Autodesk Inventor part; units mm, degrees
ref_plane "YZ Plane" through (0, 0, 0) normal (1, 0, 0) x (0, 1, 0)
ref_plane "XZ Plane" through (0, 0, 0) normal (0, 1, 0) x (-1, 0, 0)
ref_plane "XY Plane" through (0, 0, 0) normal (0, 0, 1) x (1, 0, 0)
sketch "Sketch1" plane through (0, 0, 0) normal (0, 1, 0) x (-1, 0, 0)
  circle A0 centre (0, 0) radius 1.905
  dimension "d0" = 3.81
extrude "Extrusion1" add sketch "Sketch1" along normal blind 9.9314
thread "Thread1"
sketch "Sketch2" plane through (0, 9.9314, 0) normal (0, 1, 0) x (1, 0, 0)
  line L0 (0, -3.4544) -> (-2.9916, -1.7272)
  line L1 (-2.9916, -1.7272) -> (-2.9916, 1.7272)
  line L2 (-2.9916, 1.7272) -> (0, 3.4544)
  line L3 (0, 3.4544) -> (2.9916, 1.7272)
  line L4 (2.9916, 1.7272) -> (2.9916, -1.7272)
  line L5 (2.9916, -1.7272) -> (0, -3.4544)
  point P0 (0, 0)
  point P1 (0, 0)
  dimension "d7" = 6.9088
extrude "Extrusion2" add sketch "Sketch2" along normal blind 2.3876
fillet "Fillet1" radius 0.254 6 edges at (2.9916, 11.1252, -1.7272) (0, 11.1252, -3.4544) (-2.9916, 11.1252, -1.7272) (-2.9916, 11.1252, 1.7272) (2.9916, 11.1252, 1.7272) (0, 11.1252, 3.4544)
fillet "Fillet2" radius 0.0254 12 edges at (-2.9576, 12.319, 1.7076) (-1.4958, 12.319, 2.5908) (0, 12.319, 3.4151) (1.4958, 12.319, 2.5908) (2.9576, 12.319, 1.7076) (2.9916, 12.319, 0) (2.9576, 12.319, -1.7076) (1.4958, 12.319, -2.5908) (0, 12.319, -3.4151) (-1.4958, 12.319, -2.5908) (-2.9576, 12.319, -1.7076) (-2.9916, 12.319, 0)
sketch "Sketch3" plane through (0, 12.319, 0) normal (0, 1, 0) x (1, 0, 0)
  line L0 (2.54, 0.4699) -> (-2.54, 0.4699)
  line L1 (-2.54, 0.4699) -> (-2.54, -0.4699)
  line L2 (-2.54, -0.4699) -> (2.54, -0.4699)
  line L3 (2.54, -0.4699) -> (2.54, 0.4699)
  line L4 (0.4699, 2.54) -> (-0.4699, 2.54)
  line L5 (-0.4699, 2.54) -> (-0.4699, -2.54)
  line L6 (-0.4699, -2.54) -> (0.4699, -2.54)
  line L7 (0.4699, -2.54) -> (0.4699, 2.54)
  line L8 (2.9916, -1.5806) -> (2.9916, 1.5806)
  line L9 (-2.9662, -1.5806) -> (-2.9662, 1.5806)
  point P0 (0, 0)
  point P1 (2.54, 0)
  point P2 (-0.4699, 0)
  point P3 (0, -2.54)
  point P4 (0, -0.4699)
  dimension "d12" = 0.9398
  dimension "d13" = 0.9398
  dimension "d14" = 5.08
  dimension "d15" = 5.08
  dimension "d16" = 0.4516
  dimension "d17" = 0.4262
extrude "Extrusion3" cut sketch "Sketch3" against normal blind 1.8796
chamfer "Chamfer1" distance 0.2032 angle 45 12 edges at (-1.505, 12.319, -0.4699) (-1.505, 12.319, 0.4699) (-2.54, 12.319, 0) (-0.4699, 12.319, -1.505) (0, 12.319, -2.54) (0.4699, 12.319, -1.505) (1.505, 12.319, -0.4699) (2.54, 12.319, 0) (1.505, 12.319, 0.4699) (0.4699, 12.319, 1.505) (0, 12.319, 2.54) (-0.4699, 12.319, 1.505)
chamfer "Chamfer2" distance 0.2032 angle 45 4 edges at (-0.5715, 12.2174, -0.5715) (0.5715, 12.2174, -0.5715) (-0.5715, 12.2174, 0.5715) (0.5715, 12.2174, 0.5715)
chamfer "Chamfer3" distance 1.016 angle 45 1 edges at (2.54, 10.4394, 0)
chamfer "Chamfer4" distance 1.016 angle 45 3 edges at (0, 10.4394, 2.54) (-2.54, 10.4394, 0) (0, 10.4394, -2.54)
properties part number "SSR-40 DA Screw" material "Nickel-Copper Alloy 400"
Verification items for the finished model (mm, model axes). A direction names the side the tool comes from. Give positions to 0.01 mm unless a question says otherwise; leave off trailing zeros. Order: outer loops, then holes, each group sorted by start corner. A loop starts at its lowest first (then second) coordinate and runs counter-clockwise, first axis right, second up. Notation, with made-up numbers: M 10,13.25 L 68,13.25 A8 ccw 68,23.25 Z; hole C 65,-1.75 d1. An arc over 180 degrees is marked long. Use one line per item in the form item = value. Start each with the question number.
Q1. Section check C-C (y = 7.25). Enter the section's corners in (x, z) (3 decimals), then the cut area to 3 significant figures.
Q2. Scan lines: line 1 along Z through (x, y) = (0, 8.5) (3 decimals); line 2 along Y through (x, z) = (1.95, -2); line 3 along Z through (x, y) = (-1.2, 10.5). Record each from-to range of solid material in increasing order. Write a range as [from, to].
Q3. Section check B-B (z = 0). Enter the section's corners in (x, y) (3 decimals).
Q4. Mould release check, pull along Z, two halves, no side actions. Record for faces 1 (the flat face through (-0.47, 11, -1)), 2 (the flat face through (0, 0, 0)), 3 (the flat face through (-1.515, 11.096, -2.58)): +Z half, -Z half, draft (parallel to the pull), parting line (faces both ways), or undercut.
Q5. Go/stop test with flat-tipped pins: pin 1 Ø0.5 at (x, y) = (-1.5, 11) entering from -Z; pin 2 Ø0.8 at (x, y) = (1, 11) entering from -Z; pin 3 Ø3 at (x, y) = (1, 8) entering from -Z (3 decimals). Record where each tip stops, or that it passes through.
Q6. Section check A-A (y = 10.25). Enter the section's corners in (x, z), then the cut area to 3 significant figures.
Q7. Access from +Z, -Z, +X, -X, +Y, -Y to the whole of each face (thin tool, end or side, straight path). Record for faces 4 (the flat face through (-0.47, 11, 1)), 5 (the flat face through (2.992, 11, 0)), 6 (the flat face through (2, 9.931, 1)).
Evaluation:
q1.outline = C 0,0 d3.81
q1.area = 11.4 mm2
q2.line_1 = [-1.905, 1.905]
q2.line_2 = [9.93, 12.32]
q2.line_3 = [-2.76, -0.47], [0.47, 2.76]
q3.outline = M -2.992,9.931 L -1.905,9.931 L -1.905,0 L 1.905,0 L 1.905,9.931 L 2.992,9.931 L 2.992,12.294 A0.025 ccw 2.966,12.319 L 2.743,12.319 L 2.54,12.116 L 2.54,11.455 L 1.524,10.439 L -1.524,10.439 L -2.54,11.455 L -2.54,12.116 L -2.743,12.319 L -2.966,12.319 A0.025 ccw -2.992,12.294 Z
q4.face_1 = undercut
q4.face_2 = draft
q4.face_3 = -Z half
q5.pin_1 = -2.73
q5.pin_2 = -3.11
q5.pin_3 = -1.905
q6.outline = M -2.99,-1.58 A0.25 ccw -2.86,-1.8 L -0.13,-3.38 A0.25 ccw 0.13,-3.38 L 2.86,-1.8 A0.25 ccw 2.99,-1.58 L 2.99,1.58 A0.25 ccw 2.86,1.8 L 0.13,3.38 A0.25 ccw -0.13,3.38 L -2.86,1.8 A0.25 ccw -2.99,1.58 Z
q6.area = 31.0 mm2
q7.face_4 = +Y
q7.face_5 = +Z, -Z, +X, +Y, -Y
q7.face_6 = -Y
